from build123d import *

# Parameters (mm, degrees)
SKETCH1_R           = 1.984375
BOSS_EXTRUDE1_DEPTH = 3.175


with BuildPart() as part:
    # Sketch1 → Boss-Extrude1 (new body)
    with BuildSketch(Plane(origin=(0, 0, 0), x_dir=(1, 0, 0), z_dir=(0, 1, 0))):
        Polygon((-12.7, 101.6), (12.7, 101.6), (63.5, 25.4), (63.5, 0), (-63.5, 0), (-63.5, 25.4), align=None)
        with Locations(Location((6.35, 88.9, 0), (0, 0, 270))):
            Circle(SKETCH1_R, mode=Mode.SUBTRACT)
        with Locations(Location((6.35, 63.5, 0), (0, 0, 270))):
            Circle(SKETCH1_R, mode=Mode.SUBTRACT)
        with Locations(Location((6.35, 38.1, 0), (0, 0, 270))):
            Circle(SKETCH1_R, mode=Mode.SUBTRACT)
        with Locations(Location((12.7, 12.7, 0), (0, 0, 270))):
            Circle(SKETCH1_R, mode=Mode.SUBTRACT)
        with Locations(Location((25.4, 6.35, 0), (0, 0, 270))):
            Circle(SKETCH1_R, mode=Mode.SUBTRACT)
        with Locations(Location((25.4, 19.05, 0), (0, 0, 270))):
            Circle(SKETCH1_R, mode=Mode.SUBTRACT)
        with Locations(Location((38.1, 12.7, 0), (0, 0, 270))):
            Circle(SKETCH1_R, mode=Mode.SUBTRACT)
        with Locations(Location((50.8, 6.35, 0), (0, 0, 270))):
            Circle(SKETCH1_R, mode=Mode.SUBTRACT)
        with Locations(Location((50.8, 19.05, 0), (0, 0, 270))):
            Circle(SKETCH1_R, mode=Mode.SUBTRACT)
        with Locations(Location((0, 76.2, 0), (0, 0, 90))):
            Circle(SKETCH1_R, mode=Mode.SUBTRACT)
        with Locations(Location((0, 50.8, 0), (0, 0, 90))):
            Circle(SKETCH1_R, mode=Mode.SUBTRACT)
        with Locations(Location((0, 19.05, 0), (0, 0, 90))):
            Circle(SKETCH1_R, mode=Mode.SUBTRACT)
        with Locations(Location((0, 6.35, 0), (0, 0, 90))):
            Circle(SKETCH1_R, mode=Mode.SUBTRACT)
        with Locations(Location((-50.8, 19.05, 0), (0, 0, 90))):
            Circle(SKETCH1_R, mode=Mode.SUBTRACT)
        with Locations(Location((-50.8, 6.35, 0), (0, 0, 90))):
            Circle(SKETCH1_R, mode=Mode.SUBTRACT)
        with Locations(Location((-38.1, 12.7, 0), (0, 0, 90))):
            Circle(SKETCH1_R, mode=Mode.SUBTRACT)
        with Locations(Location((-25.4, 19.05, 0), (0, 0, 90))):
            Circle(SKETCH1_R, mode=Mode.SUBTRACT)
        with Locations(Location((-25.4, 6.35, 0), (0, 0, 90))):
            Circle(SKETCH1_R, mode=Mode.SUBTRACT)
        with Locations(Location((-12.7, 12.7, 0), (0, 0, 90))):
            Circle(SKETCH1_R, mode=Mode.SUBTRACT)
        with Locations(Location((-6.35, 38.1, 0), (0, 0, 90))):
            Circle(SKETCH1_R, mode=Mode.SUBTRACT)
        with Locations(Location((-6.35, 63.5, 0), (0, 0, 90))):
            Circle(SKETCH1_R, mode=Mode.SUBTRACT)
        with Locations(Location((-6.35, 88.9, 0), (0, 0, 90))):
            Circle(SKETCH1_R, mode=Mode.SUBTRACT)
    extrude(amount=BOSS_EXTRUDE1_DEPTH)


solid = part.part
Design review of the part built by this model. Coordinates are the model's own, in mm. Coordinates: 2 decimals unless noted, no trailing zeros. Order: outer loops, then holes, each group sorted by start corner. A loop starts at its lowest first (then second) coordinate and runs counter-clockwise, first axis right, second up. Notation, with made-up numbers: (-1.75, 20.5) - (16.25, 20.5) arc R25 ccw to (16.25, 38.5) - close; hole circle Ø6 at (22, 71.25). An arc over 180 degrees is marked (long way). Put each result on its own line as item: value.
1) The part is to be moulded in two halves that separate along Z. For faces 1 (the face through (-5.59, 1.565, -65.333)), 2 (the face through (1, 0, -40)), 3 (the face through (-38.456, 1.565, -62.967)), say which applies: released by +Z, released by -Z, zero draft, split by the parting line, or undercut.
Response values:
face 1: undercut
face 2: zero draft
face 3: released by -Z
2) Take a section at C-C, the plane x = 50.8. Give the boundary of the cut face in (y, z) (3 decimals).
Response values:
outline: (0, -44.45) - (3.175, -44.45) - (3.175, -21.034) - (0, -21.034) - close; (0, -17.066) - (3.175, -17.066) - (3.175, -8.334) - (0, -8.334) - close; (0, -4.366) - (3.175, -4.366) - (3.175, 0) - (0, 0) - close
3) Take a section at B-B, the plane y = 2.55. Count the separate pieces of the cut face and the enclosed holes in it, and give its area (3 significant figures).
Response values:
separate pieces: 1
enclosed holes: 22
area: 8,760 mm²
4) Take a section at D-D, the plane z = -12.7. Give the boundary of the cut face in (x, y) (3 decimals), and give its area (3 significant figures).
Response values:
outline: (-63.5, 0) - (-40.084, 0) - (-40.084, 3.175) - (-63.5, 3.175) - close; (-36.116, 0) - (-14.684, 0) - (-14.684, 3.175) - (-36.116, 3.175) - close; (-10.716, 0) - (10.716, 0) - (10.716, 3.175) - (-10.716, 3.175) - close; (14.684, 0) - (36.116, 0) - (36.116, 3.175) - (14.684, 3.175) - close; (40.084, 0) - (63.5, 0) - (63.5, 3.175) - (40.084, 3.175) - close
area: 353 mm²
5) Wall thickness on L1, parallel to X at y = 1, z = -19.05; L2, parallel to Z at x = -0.5, y = 1.3; L3, parallel to Z at x = -50.8, y = 1.65: over which ranges is each line inside the solid? List them lowest first. Write a range as from..to.
Response values:
L1: x = -63.5..-52.78, -48.82..-27.38, -23.42..-1.98, 1.98..23.42, 27.38..48.82, 52.78..63.5
L2: z = -101.6..-78.12, -74.28..-52.72, -48.88..-20.97, -17.13..-8.27, -4.43..0
L3: z = -44.45..-21.03, -17.07..-8.33, -4.37..0
6) Take a section at A-A, the plane x = 0. Give the boundary of the cut face in (y, z) (3 decimals), and give its area (3 significant figures).
Response values:
outline: (0, -101.6) - (3.175, -101.6) - (3.175, -78.184) - (0, -78.184) - close; (0, -74.216) - (3.175, -74.216) - (3.175, -52.784) - (0, -52.784) - close; (0, -48.816) - (3.175, -48.816) - (3.175, -21.034) - (0, -21.034) - close; (0, -17.066) - (3.175, -17.066) - (3.175, -8.334) - (0, -8.334) - close; (0, -4.366) - (3.175, -4.366) - (3.175, 0) - (0, 0) - close
area: 272 mm²
7) Insertion check: P1, Ø3, axis at x = 6.35, z = -63.5, coming from the -Y side; P2, Ø1, axis at y = 2, z = -55.5, coming from the +X side; P3, Ø1, axis at x = -37.5, y = 1, coming from the -Z side. Each pin has a flat end and moves straight along its axis. Give the tip position at first contact, or say it passes through.
Response values:
P1: passes through
P2: stops at x = 43.77
P3: stops at z = -65.15
